Here's how the part is built. I have some questions about the finished solid (model axes, mm). A direction names the side the tool comes from. Round coordinates to 2 decimals unless told otherwise and drop trailing zeros. Write each loop counter-clockwise with the first axis right and the second up, starting at its lowest first coordinate (ties: lowest second). Pieces come first, ordered by that corner, then holes. Notation, with made-up numbers: (48.25, 11) - (69.25, 11) arc R22 ccw to (69.25, 24) - close; hole circle Ø7 at (0, -22.75). An arc over 180 degrees is marked (long way). One line per item, written item: value. Start each with the question number.
Item 1: If I drill on line 1 (Z direction, x = -207.5, y = 45); line 2 (X direction, y = 58.5, z = -128); line 3 (Y direction, x = 31, z = -11.5), over which ranges is the centre line in solid material (lowest first)?
Item 2: Thinking about a two-plate mould opening in Z: for faces 1 (the face through (243.7, 61.1, 150.8)), 2 (the face through (229.244, 71.272, -136.972)), 3 (the face through (-4, 0, -2)), which applies, released by +Z, released by -Z, zero draft, split by the parting line, or undercut?
Item 3: Imagine slicing it at B-B, the plane y = 75. Please give me the cut outline in (x, z).
Item 4: For P1, Ø1.5, axis at x = -128, z = -70.5, coming from the +Y side, with a flat end and sliding along its axis, tell me the tip position at first contact or that it passes through.
Item 5: Imagine slicing it at A-A, the plane x = -201.5. Please give me the cut outline in (y, z).
Item 6: Imagine slicing it at C-C, the plane z = -73.5. Please give me the cut outline in (x, y), then the cut area to 3 significant figures.
Item 7: For faces 4 (the face through (-257.5, 61, 2)), 5 (the face through (-3, 20, -2)), which set-ups out of +Z, -Z, +X, -X, +Y, -Y let a thin tool reach every point of the face, with its end or its side?
```python
from build123d import *

# Parameters (mm, degrees)
SKETCH1_W           = 515
SKETCH1_H           = 330
BOSS_EXTRUDE1_DEPTH = 124
CHAMFER1_SIZE       = 28
SHELL1_T            = -20


with BuildPart() as part:
    # Sketch1 → Boss-Extrude1 (new body)
    with BuildSketch(Plane(origin=(0, 0, 0), x_dir=(1, 0, 0), z_dir=(0, 1, 0))):
        Rectangle(SKETCH1_W, SKETCH1_H)
    extrude(amount=BOSS_EXTRUDE1_DEPTH)

    # Chamfer1
    chamfer1_edges = [part.edges().sort_by_distance(p)[0] for p in [
        (257.5, 62, 165),
        (-257.5, 62, 165),
        (-257.5, 62, -165),
        (257.5, 62, -165),
    ]]
    chamfer(chamfer1_edges, length=CHAMFER1_SIZE)

    # Shell1
    shell1_openings = [part.faces().sort_by_distance(p)[0] for p in [
        (0, 124, 0),
    ]]
    offset(amount=SHELL1_T, openings=shell1_openings, kind=Kind.INTERSECTION)


solid = part.part
```
Values follow:
1. line 1: z = -165 to -145, 145 to 165
1. line 2: x = -257.5 to -237.5, 237.5 to 257.5
1. line 3: y = 0 to 20
2. face 1: released by +Z
2. face 2: undercut
2. face 3: zero draft
3. outline: (-257.5, -137) - (-229.5, -165) - (229.5, -165) - (257.5, -137) - (257.5, 137) - (229.5, 165) - (-229.5, 165) - (-257.5, 137) - close; hole (-237.5, -128.72) - (-221.22, -145) - (221.22, -145) - (237.5, -128.72) - (237.5, 128.72) - (221.22, 145) - (-221.22, 145) - (-237.5, 128.72) - close
4. P1: stops at y = 20
5. outline: (0, -165) - (124, -165) - (124, -145) - (20, -145) - (20, 145) - (124, 145) - (124, 165) - (0, 165) - close
6. outline: (-257.5, 0) - (257.5, 0) - (257.5, 124) - (237.5, 124) - (237.5, 20) - (-237.5, 20) - (-237.5, 124) - (-257.5, 124) - close
6. area: 14,500 mm^2
7. face 4: +Z, -Z, -X, +Y, -Y
7. face 5: +Y
